from build123d import *

# Parameters (mm, degrees)
F0_W     = 20
F0_H     = 30
F1_DEPTH = 3
F2_R     = 5
F3_DEPTH = 10
F6_R     = 5


with BuildPart() as f1:
    # F0 (on Top) → F1 (new body)
    with BuildSketch(Plane.XY):
        Rectangle(F0_W, F0_H)
    extrude(amount=F1_DEPTH)

    # F2 (on face) → F3 (join)
    with BuildSketch(Plane.XY.offset(3)):
        Circle(F2_R)
    extrude(amount=F3_DEPTH)

    # F9: sweep along a path in F8
    with BuildLine(Plane.YZ) as f9_path:
        Line((0, 13), (7, 23))
    # F6 (on face) → F9 (sweep)
    with BuildSketch(Plane.XY.offset(13)):
        Circle(F6_R)
    sweep(path=f9_path.line)


solid = f1.part
Input: part model. Units: mm. Frame: model coordinates. A direction names the side the tool comes from. Round coordinates to 2 decimals unless told otherwise and drop trailing zeros. Write each loop counter-clockwise with the first axis right and the second up, starting at its lowest first coordinate (ties: lowest second). Pieces come first, ordered by that corner, then holes.
1) Ray query, L1, parallel to Z at x = -8, y = -5.5; L2, parallel to Z at x = -1.25, y = 0; L3, parallel to X at y = -1, z = 4.25. Return the intervals inside material, ascending.
2) Reachability of faces 1 (the cylindrical face through (-1.08, -4.88, 7.93)), 2 (the flat face through (0, 15, 1)) from +Z, -Z, +X, -X, +Y, -Y: full face, straight path, thin tool, end or side. Return the list, or none.
3) Draft query along Z for faces 3 (the flat face through (0, -15, 1)), 4 (the flat face through (0, 7, 23)), 5 (the flat face through (4, 4, 3)). Return one class per face: pulls with the +Z half, pulls with the -Z half, needs draft (parallel to the pull), parting line crosses it, or undercut.
4) Cut plane A-A (x = 6). Return the cut outline in (y, z), then the cut area to 3 significant figures.
5) Contact query for flat-ended pins moving along their axis: P1, Ø4, axis at x = 5, z = 9.5, coming from the -Y side; P2, Ø10, axis at y = -6, z = 11, coming from the -X side; P3, Ø12, axis at y = 3.5, z = 9.5, coming from the -X side. Output: stop coordinate, or through.
Geometry says:
1. L1: z = 0 to 3
1. L2: z = 0 to 19.92
1. L3: x = -4.9 to 4.9
2. face 1: none
2. face 2: +Z, -Z, +X, -X, +Y
3. face 3: needs draft
3. face 4: pulls with the +Z half
3. face 5: undercut
4. outline: (-15, 0) - (15, 0) - (15, 3) - (-15, 3) - close
4. area: 90.0 mm2
5. P1: stops at y = -4
5. P2: stops at x = -4.9
5. P3: stops at x = -5
